For this review, take the finished solid that the model builds, in its own axes (mm). Face numbers are marked on the shaded views. A direction names the side the tool comes from. Round coordinates to 2 decimals unless told otherwise and drop trailing zeros. Loops run counter-clockwise (first coordinate to the right, second up) from the corner with the lowest first, then second, coordinate; pieces in that order, holes last. Notation, with made-up numbers: M 23.25,42.25 L 60.25,42.25 A26 cw 60.25,61.25 Z; hole C 35.5,-17 d5. An arc over 180 degrees is marked long. One line per question, with ' | ' between items. Start each with the question number.
1) We need section A-A (z = -4.25). Give the boundary of the cut face in (x, y).
2) We need section B-B (y = -30). Give the boundary of the cut face in (x, z).
3) We need section C-C (y = -7). Give the boundary of the cut face in (x, z).
4) We need section D-D (z = 4.5). Give the boundary of the cut face in (x, y), and give its area (3 significant figures).
5) For probe 1 along Y at (x, z) = (0, -2); probe 2 along Z at (x, y) = (10.65, -30); probe 3 along Y at (x, z) = (8, 2.5), list the stretches that pass through material, from the lowest coordinate up. Write a range as from..to.
6) For the marked faces 1 and 2, list the 3-axis set-ups (+Z, -Z, +X, -X, +Y, -Y) from which the entire face can be reached by the end or side of a thin tool; tool diameter is ignored.
7) For pin 1 Ø2.5 at (y, z) = (-30, 0) entering from +X; pin 2 Ø8 at (x, y) = (4.5, -5) entering from -Z; pin 3 Ø2 at (y, z) = (-30, 0.5) entering from -X, all flat-tipped, find the tip position at first contact; note any pin that passes through.
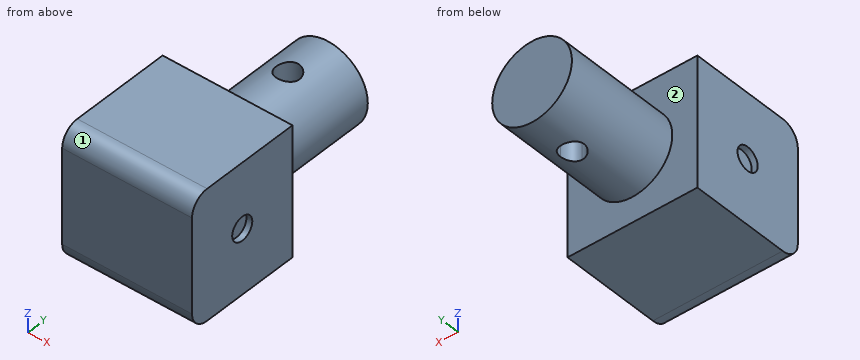
```python
from build123d import *

# Parameters (mm, degrees)
F0_R      = 6.75
F1_DEPTH  = 20
F2_W      = 22
F2_H      = 22
F3_DEPTH  = 20
F4_R      = 3
F6_DEPTH  = 1
F7_R      = 2
F8_DEPTH  = 1
F10_DEPTH = 25


with BuildPart() as f1:
    # F0 (on Front) → F1 (new body)
    with BuildSketch(Plane.XZ):
        Circle(F0_R)
    extrude(amount=F1_DEPTH)

    # F2 (on face) → F3 (join)
    with BuildSketch(Plane.XZ.offset(20)):
        Rectangle(F2_W, F2_H)
    extrude(amount=F3_DEPTH)

    # F4
    f4_edges = [f1.edges().sort_by_distance(p)[0] for p in [
        (0, -40, 11),
        (0, -40, -11),
    ]]
    fillet(f4_edges, radius=F4_R)

    # F5 (on face) → F6 (cut)
    with BuildSketch(Plane.YZ.offset(11)):
        with BuildLine():
            ThreePointArc((-32, 0), (-30, -2), (-28, 0))
            ThreePointArc((-28, 0), (-30, 2), (-32, 0))
        make_face()
    extrude(amount=-F6_DEPTH, mode=Mode.SUBTRACT)

    # F7 (on face) → F8 (cut)
    with BuildSketch(Plane(origin=(-11, 0, 0), x_dir=(0, -1, 0), z_dir=(-1, 0, 0))):
        with Locations((30, 0)):
            Circle(F7_R)
    extrude(amount=-F8_DEPTH, mode=Mode.SUBTRACT)

    # F9 (on face) → F10 (cut)
    with BuildSketch(Plane.XY.offset(11)):
        with BuildLine():
            ThreePointArc((2, -8), (-1.414214, -6.585786), (0, -10))
            ThreePointArc((0, -10), (1.414214, -9.414214), (2, -8))
        make_face()
    extrude(amount=-F10_DEPTH, mode=Mode.SUBTRACT)


solid = f1.part
```
Answers below:
1) outline: M -11,-40 L 11,-40 L 11,-20 L 5.24,-20 L 5.24,0 L -5.24,0 L -5.24,-20 L -11,-20 Z; hole M 0,-10 A2 ccw 2,-8 A2 ccw long Z
2) outline: M -11,-11 L 11,-11 L 11,-2 L 10,-2 L 10,2 L 11,2 L 11,11 L -11,11 L -11,2 L -10,2 L -10,-2 L -11,-2 Z
3) outline: M -1.73,-6.52 L -1.73,6.52 A6.75 ccw Z; M 1.73,-6.52 A6.75 ccw 1.73,6.52 Z
4) outline: M -11,-40 L 11,-40 L 11,-20 L 5.03,-20 L 5.03,0 L -5.03,0 L -5.03,-20 L -11,-20 Z; hole M 0,-10 A2 ccw 2,-8 A2 ccw long Z | area: 629 mm^2
5) probe 1: -40..-10, -6..0 | probe 2: -11..-2, 2..11 | probe 3: -40..-20
6) face 1: +Z, +X, -X, -Y | face 2: +Y
7) pin 1: x = 10 | pin 2: z = -6.73 | pin 3: x = -10
